Read the model definition and answer for the solid it produces. Units are mm, in the model's axes. A direction names the side the tool comes from. Round coordinates to 2 decimals unless told otherwise and drop trailing zeros. Order: outer loops, then holes, each group sorted by start corner. A loop starts at its lowest first (then second) coordinate and runs counter-clockwise, first axis right, second up.
from build123d import *

# Parameters (mm, degrees)
SKETCH1_R           = 6.35
BOSS_EXTRUDE3_DEPTH = 12.7


with BuildPart() as part:
    # Sketch1 → Boss-Extrude3 (new body)
    with BuildSketch(Plane.XY):
        with BuildLine():
            Line((-12.7, -336.612), (-12.7, -350))
            ThreePointArc((-12.7, -350), (0, -362.7), (12.7, -350))
            Line((12.7, -350), (12.7, 0))
            ThreePointArc((12.7, 0), (0, 12.7), (-12.7, 0))
            Line((-12.7, 0), (-12.7, -287.212))
            ThreePointArc((-12.7, -287.212), (-16.214718626, -295.697281374), (-24.7, -299.212))
            Line((-24.7, -299.212), (-57.15, -299.212))
            ThreePointArc((-57.15, -299.212), (-69.85, -311.912), (-57.15, -324.612))
            Line((-57.15, -324.612), (-24.7, -324.612))
            ThreePointArc((-24.7, -324.612), (-16.214718626, -328.126718626), (-12.7, -336.612))
        make_face()
        Circle(SKETCH1_R, mode=Mode.SUBTRACT)
        with Locations((-57.15, -311.912)):
            Circle(SKETCH1_R, mode=Mode.SUBTRACT)
        with Locations((0, -350)):
            Circle(SKETCH1_R, mode=Mode.SUBTRACT)
    extrude(amount=BOSS_EXTRUDE3_DEPTH)


solid = part.part
Q1. Flat-ended cylindrical pins translate along their axes: pin 1 (6.5 mm diameter, centred on x = -37.5, z = 9, fed in from -Y); pin 2 (1 mm diameter, centred on x = -3, z = 7, fed in from +Y); pin 3 (6.5 mm diameter, centred on x = -40.5, z = 5.5, fed in from +Y). Find the tip coordinate at first contact, or state that the pin passes through.
Outcome:
pin 1: stops at y = -324.61
pin 2: stops at y = 12.45
pin 3: stops at y = -299.21
Q2. A cutting plane is placed at D-D, the plane y = -294. Give the vertices of the cut face in (x, z), plus the area to 3 significant figures.
Outcome:
outline: (-14.8, 0) - (12.7, 0) - (12.7, 12.7) - (-14.8, 12.7) - close
area: 349 mm2
Q3. A cutting plane is placed at A-A, the plane x = 0. Give the vertices of the cut face in (y, z), plus the area to 4 significant figures.
Outcome:
outline: (-362.7, 0) - (-356.35, 0) - (-356.35, 12.7) - (-362.7, 12.7) - close; (-343.65, 0) - (-6.35, 0) - (-6.35, 12.7) - (-343.65, 12.7) - close; (6.35, 0) - (12.7, 0) - (12.7, 12.7) - (6.35, 12.7) - close
area: 4,445 mm2
Q4. A cutting plane is placed at C-C, the plane y = -34. Give the vertices of the cut face in (x, z), plus the area to 3 significant figures.
Outcome:
outline: (-12.7, 0) - (12.7, 0) - (12.7, 12.7) - (-12.7, 12.7) - close
area: 323 mm2
Q5. A cutting plane is placed at B-B, the plane z = 8.25. Give the vertices of the cut face in (x, y).
Outcome:
outline: (-57.15, -324.61) - (-24.7, -324.61) arc R12 cw to (-12.7, -336.61) - (-12.7, -350) arc R12.7 ccw to (12.7, -350) - (12.7, 0) arc R12.7 ccw to (-12.7, 0) - (-12.7, -287.21) arc R12 cw to (-24.7, -299.21) - (-57.15, -299.21) arc R12.7 ccw to start; hole circle Ø12.7 at (-57.15, -311.91); hole circle Ø12.7 at (0, -350); hole circle Ø12.7 at (0, 0)
Q6. For faces 5 (the face through (-41, -299.212, 6)), 6 (the face through (-0.279, -362.697, 6.261)), determine the directions among +Z, -Z, +X, -X, +Y, -Y from which every point of the face is accessible in a straight line to the end or side of a thin tool.
Outcome:
face 5: +Z, -Z, -X, +Y
face 6: +Z, -Z, -Y
Q7. Straight lines are drawn through the part: probe 1 along Y at (x, z) = (0, 4.25); probe 2 along X at (y, z) = (-350, 4); probe 3 along Y at (x, z) = (-57.15, 6.75). For each, find the intervals that lie inside material, in ascending order.
Outcome:
probe 1: y = -362.7 to -356.35, -343.65 to -6.35, 6.35 to 12.7
probe 2: x = -12.7 to -6.35, 6.35 to 12.7
probe 3: y = -324.61 to -318.26, -305.56 to -299.21
Q8. For a pull along Y with two mould halves and no side action, classify faces 1 (the face through (-12.7, -343, 6)), 2 (the face through (-41, -324.612, 6)), 3 (the face through (-1.38, -6.2, 6.26)), 4 (the face through (-16.12, -295.6, 6.26)) as released by +Y, released by -Y, zero draft, split by the parting line, or undercut.
Outcome:
face 1: zero draft
face 2: released by -Y
face 3: undercut
face 4: released by +Y
